Could you check a few things on this drawing? It's one solid part, dimensions in mm from its lowest x, y, z. A direction names the side the tool comes from. Round coordinates to 2 decimals unless told otherwise and drop trailing zeros. Loops run counter-clockwise (first coordinate to the right, second up) from the corner with the lowest first, then second, coordinate; pieces in that order, holes last. Notation, with made-up numbers: M -18,27.25 L 36,27.25 A23 cw 36,54.25 Z; hole C 78.5,51 d8. An arc over 180 degrees is marked long. Return JSON: item names as keys, results as strings.
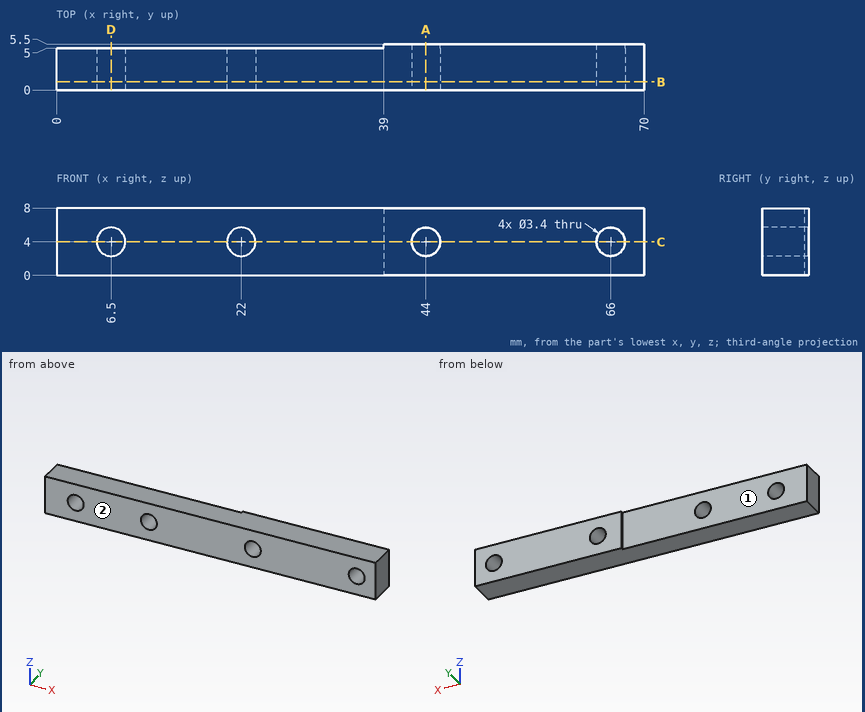
Q1. Suppose I cut it at B-B, the plane y = 1. Please give me the cut outline in (x, z).
Results:
{"outline": "M 0,0 L 70,0 L 70,8 L 0,8 Z; hole C 6.5,4 d3.4; hole C 22,4 d3.4; hole C 44,4 d3.4; hole C 66,4 d3.4"}
Q2. I'm going to push flat-ended pins straight in: pin 1 Ø1 at (x, z) = (16, 3) entering from +Y; pin 2 Ø0.6 at (y, z) = (5, 2) entering from -X; pin 3 Ø3 at (x, z) = (22, 4) entering from -Y. Where does each tip first touch, or does it pass through?
Results:
{"pin 1": "stops at y = 5", "pin 2": "stops at x = 0", "pin 3": "passes through"}
Q3. If I drill on line 1 along X through (y, z) = (3.15, 4); line 2 along Z through (x, y) = (6.5, 1.55); line 3 along X through (y, z) = (0.65, 2.5), over which ranges is the centre line in solid material (lowest first)?
Results:
{"line 1": "x = 0 to 4.8, 8.2 to 20.3, 23.7 to 42.3, 45.7 to 64.3, 67.7 to 70", "line 2": "z = 0 to 2.3, 5.7 to 8", "line 3": "x = 0 to 5.7, 7.3 to 21.2, 22.8 to 43.2, 44.8 to 65.2, 66.8 to 70"}
Q4. Suppose I cut it at D-D, the plane x = 6.5. Please give me the cut outline in (y, z), plus the area to 3 significant figures.
Results:
{"outline": "M 0,0 L 5,0 L 5,2.3 L 0,2.3 Z; M 0,5.7 L 5,5.7 L 5,8 L 0,8 Z", "area": "23.0 mm2"}
Q5. Suppose I cut it at A-A, the plane x = 44. Please give me the cut outline in (y, z), plus the area to 3 significant figures.
Results:
{"outline": "M 0,0 L 5.5,0 L 5.5,2.3 L 0,2.3 Z; M 0,5.7 L 5.5,5.7 L 5.5,8 L 0,8 Z", "area": "25.3 mm2"}
Q6. Suppose I cut it at C-C, the plane z = 4. Please give me the cut outline in (x, y).
Results:
{"outline": "M 0,0 L 4.8,0 L 4.8,5 L 0,5 Z; M 8.2,0 L 20.3,0 L 20.3,5 L 8.2,5 Z; M 23.7,0 L 42.3,0 L 42.3,5.5 L 39,5.5 L 39,5 L 23.7,5 Z; M 45.7,0 L 64.3,0 L 64.3,5.5 L 45.7,5.5 Z; M 67.7,0 L 70,0 L 70,5.5 L 67.7,5.5 Z"}
Q7. On a 3-axis mill with a long thin cutter (end or side, diameter ignored), from which of +Z, -Z, +X, -X, +Y, -Y can I reach the whole of each face in a straight line? I mean the marked faces 1 and 2. Say none if no direction works.
Results:
{"face 1": "+Z, -Z, -X, +Y", "face 2": "+Z, -Z, +X, -X, -Y"}
